Autodesk Inventor part; units mm, degrees
ref_plane "YZ Plane" through (0, 0, 0) normal (1, 0, 0) x (0, 1, 0)
ref_plane "XZ Plane" through (0, 0, 0) normal (0, 1, 0) x (-1, 0, 0)
ref_plane "XY Plane" through (0, 0, 0) normal (0, 0, 1) x (1, 0, 0)
sketch "Sketch1" plane through (0, 0, 0) normal (1, 0, 0) x (0, 1, 0)
  arc A0 (0, 49) -> (0, 41) centre (0, 45) ccw
  arc A1 (-1.4037, -41.2544) -> (-2.6656, -47.9824) centre (0, -45) ccw
  circle A2 centre (0, 45) radius 4
  circle A3 centre (0, -45) radius 4
  line L0 (5, 81.5) -> (-8, 81.5)
  line L1 (5, -81.5) -> (-8, -81.5)
  line L2 (5, -40) -> (-8, -40)
  line L3 (5, 40) -> (-8, 40)
  line L4 (5, 81.5) -> (5, 40)
  line L5 (5, -40) -> (5, -81.5)
  line L6 (-8, 81.5) -> (-8, 40)
  line L7 (-8, -40) -> (-8, -81.5)
  line L8 (-8, -40) -> (-13, -35.203)
  line L9 (-13, -35.203) -> (-13, 35.203)
  line L10 (-13, 35.203) -> (-8, 40)
  line L11 (5, 40) -> (-3, 32.3248)
  line L12 (-3, 32.3248) -> (-3, -32.3248)
  line L13 (-3, -32.3248) -> (5, -40)
  point P0 (0, 0)
  point P1 (0, 0)
  point P2 (-4, 45)
  point P3 (-8, -60.75)
  point P4 (-8, 60.75)
  point P5 (5, 60.75)
  dimension "d0" = 8
  dimension "d1" = 8
  dimension "d2" = 90
  dimension "d3" = 45
  dimension "d34" = 36.5
  dimension "d35" = 36.5
  dimension "d36" = 5
  dimension "d38" = 5
  dimension "d39" = 5
  dimension "d41" = 5
  dimension "d43" = 13
  dimension "d44" = 10
  dimension "d45" = 9
  dimension "d48" = 13
extrude "Extrusion1" add sketch "Sketch1" along normal blind 18
sketch "Sketch3" plane through (0, 5, 81.5) normal (0, 1, 0) x (1, 0, 0)
  circle A0 centre (9, 9) radius 4
  circle A1 centre (9, 154) radius 4
  line L0 (0, 41.5) -> (0, 0)
  line L1 (0, 0) -> (18, 0)
  line L2 (0, 163) -> (18, 163)
  point P0 (0, 81.5)
  dimension "d17" = 8
  dimension "d18" = 8
  dimension "d19" = 9
  dimension "d20" = 9
  dimension "d21" = 9
extrude "Extrusion3" cut sketch "Sketch3" against normal blind 27.75
fillet "Fillet1" radius 6 8 edges at (9, -8, -40) (9, -13, -35.203) (9, -13, 35.203) (9, -8, 40) (9, 5, -40) (9, -3, -32.3248) (9, -3, 32.3248) (9, 5, 40)
sketch "Sketch5" plane through (0, -3, 29.7664) normal (0, 1, 0) x (1, 0, 0)
  line L0 (6, 54.5327) -> (12, 54.5327)
  line L1 (12, 54.5327) -> (12, 5)
  line L2 (12, 5) -> (6, 5)
  line L3 (6, 5) -> (6, 54.5327)
  line L4 (0, 111.2664) -> (18, 111.2664)
  line L5 (0, 59.5327) -> (18, 59.5327)
  line L6 (18, 0) -> (0, 0)
  point P0 (0, 29.7664)
  point P1 (9, 54.5327)
  point P2 (9, 111.2664)
  dimension "d49" = 6
  dimension "d50" = 5
  dimension "d51" = 5
extrude "Extrusion5" cut sketch "Sketch5" against normal blind 27.75
properties part number "Frame_Mount"
Design review of the part built by this model. Coordinates are the model's own, in mm. A direction names the side the tool comes from. Round coordinates to 2 decimals unless told otherwise and drop trailing zeros. Write each loop counter-clockwise with the first axis right and the second up, starting at its lowest first coordinate (ties: lowest second). Pieces come first, ordered by that corner, then holes. Notation, with made-up numbers: (68.25, 33.25) - (108.25, 33.25) arc R23 ccw to (108.25, 43.25) - close; hole circle Ø11 at (3, 88). An arc over 180 degrees is marked (long way). Use a Markdown table: item, result. Add a question column.
1. Wall thickness on probe 1 along Z at (x, y) = (2.5, 1.75); probe 2 along Z at (x, y) = (9, 0.75); probe 3 along Z at (x, y) = (11.25, 1.5): over which ranges is each line inside the solid? List them lowest first.
2. We need section C-C (y = -5.75). State the section outline as (x, z) points, then the cut area to 3 significant figures.
3. We need section A-A (y = 0.25). State the section outline as (x, z) points.
4. Mouldability with a two-part tool opening along X and no side actions: class faces 6 (the face through (18, -4, 1)), 7 (the face through (9, -8, -24.766)), 8 (the face through (9.13, -2.53, -32.09)) as +X half, -X half, draft (parallel to the pull), parting line (faces both ways), or undercut.
5. For faces 1 (the face through (9, -8, 62)), 2 (the face through (9, -1, -81.5)), 3 (the face through (8.87, 3.95, -45.62)), 4 (the face through (9.126, -2.506, 32.151)), 5 (the face through (12, -8, 0)), list the 3-axis set-ups (+Z, -Z, +X, -X, +Y, -Y) from which the entire face can be reached by the end or side of a thin tool; tool diameter is ignored.
6. Clearance check with flat-ended pins moving along their axes: pin 1 (7 mm diameter, centred on x = 9, z = -72.5, fed in from -Y); pin 2 (10.5 mm diameter, centred on x = 9, z = 72.5, fed in from -Y); pin 3 (9 mm diameter, centred on x = 8.5, z = -10, fed in from +Y). State where each tip first meets the part, or that it passes through.
7. We need section B-B (z = 45). State the section outline as (x, y) points.
8. We need section D-D (x = 14.5). State the section outline as (y, z) points.
Output:
| question | item | result |
|---|---|---|
| 1 | probe 1 | z = -81.5 to -48.6, -41.4 to -36.88, 36.88 to 41.4, 48.6 to 81.5 |
| 1 | probe 2 | z = -81.5 to -76.5, -68.5 to -48.93, -41.07 to -35.92, 35.92 to 41.07, 48.93 to 68.5, 76.5 to 81.5 |
| 1 | probe 3 | z = -81.5 to -75.81, -69.19 to -48.71, -41.29 to -36.64, 36.64 to 41.29, 48.71 to 69.19, 75.81 to 81.5 |
| 2 | outline | (0, -81.5) - (18, -81.5) - (18, 81.5) - (0, 81.5) - close; hole circle Ø8 at (9, -72.5); hole circle Ø8 at (9, 72.5); hole (6, -24.77) - (12, -24.77) - (12, 24.77) - (6, 24.77) - close |
| 2 | area | 2,540 mm2 |
| 3 | outline | (0, -81.5) - (18, -81.5) - (18, -48.99) - (0, -48.99) - close; (0, -41.01) - (18, -41.01) - (18, -35.44) - (0, -35.44) - close; (0, 35.44) - (18, 35.44) - (18, 41.01) - (0, 41.01) - close; (0, 48.99) - (18, 48.99) - (18, 81.5) - (0, 81.5) - close; hole circle Ø8 at (9, -72.5); hole circle Ø8 at (9, 72.5) |
| 4 | face 6 | +X half |
| 4 | face 7 | undercut |
| 4 | face 8 | draft |
| 5 | face 1 | +Z, +X, -X, -Y |
| 5 | face 2 | -Z, +X, -X, +Y, -Y |
| 5 | face 3 | +X, -X |
| 5 | face 4 | +X, -X, +Y |
| 5 | face 5 | +Y, -Y |
| 6 | pin 1 | passes through |
| 6 | pin 2 | stops at y = -8 |
| 6 | pin 3 | stops at y = -3 |
| 7 | outline | (0, -8) - (18, -8) - (18, -4) - (0, -4) - close; (0, 4) - (18, 4) - (18, 5) - (0, 5) - close |
| 8 | outline | (-13, -32.64) arc R6 ccw to (-11.15, -36.97) - (-9.85, -38.23) arc R6 cw to (-8, -42.56) - (-8, -81.5) - (5, -81.5) - (5, -42.56) arc R6 ccw to (3.15, -38.23) - (-1.15, -34.1) arc R6 cw to (-3, -29.77) - (-3, 29.77) arc R6 cw to (-1.15, 34.1) - (3.15, 38.23) arc R6 ccw to (5, 42.56) - (5, 81.5) - (-8, 81.5) - (-8, 42.56) arc R6 cw to (-9.85, 38.23) - (-11.15, 36.97) arc R6 ccw to (-13, 32.64) - close; hole circle Ø8 at (0, 45); hole (-2.67, -47.98) arc R4 ccw (long way) to (-1.4, -41.25) arc R4 ccw to start |
